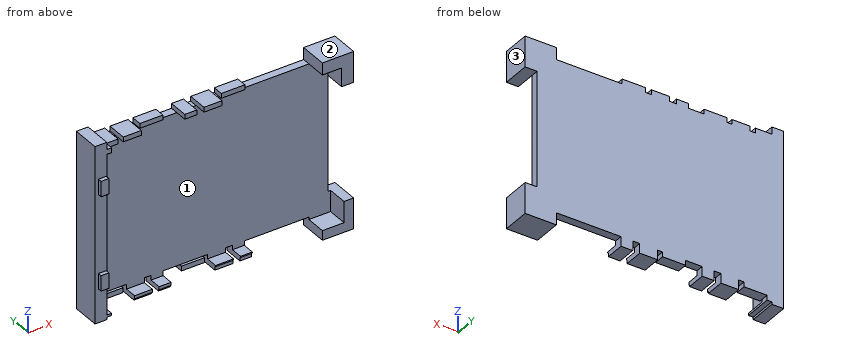
```python
from build123d import *

# Parameters (mm, degrees)
CORNERS_DEPTH                      = 8.4
CORNERS_2_DEPTH                    = 8.4
SKETCH2_W                          = 102.6
SKETCH2_H                          = 63.5
MASTER_DEPTH                       = 3
SKETCH3_W                          = 4.9
SKETCH3_H                          = 73.5
END_TAB_DEPTH                      = 8.36
END_TAB_DEPTH_BACK                 = 3.27
SKETCH4_W                          = 3.2
SKETCH4_H                          = 6.4
MALE_CONNECTORS_DEPTH              = 1.65
SKETCH5_W                          = 9.6
SKETCH5_H                          = 2
SKETCH5_W_2                        = 7.4
SKETCH5_H_2                        = 4
SKETCH5_W_3                        = 5
SKETCH5_W_4                        = 7.5
SKETCH5_W_5                        = 4.9
RIGHT_TERMINALS_DEPTH              = 5
RIGHT_TERMINALS_DEPTH_BACK         = 3.27
SKETCH7_W                          = 4.9
SKETCH7_H                          = 2
LEFT_TERMINALS_DEPTH               = 5
LEFT_TERMINALS_DEPTH_BACK          = 3.27
SKETCH7_W_2                        = 7.5
LEFT_TERMINALS_2_DEPTH             = 5
LEFT_TERMINALS_2_DEPTH_BACK        = 3.27
SKETCH7_W_3                        = 9.6
LEFT_TERMINALS_3_DEPTH             = 5
LEFT_TERMINALS_3_DEPTH_BACK        = 3.27
SKETCH7_W_4                        = 5
LEFT_TERMINALS_4_DEPTH             = 5
LEFT_TERMINALS_4_DEPTH_BACK        = 3.27
LEFT_TERMINALS_5_DEPTH             = 5
LEFT_TERMINALS_5_DEPTH_BACK        = 3.27
SKETCH7_W_5                        = 9.8
LEFT_TERMINALS_6_DEPTH             = 5
LEFT_TERMINALS_6_DEPTH_BACK        = 3.27
SKETCH8_W                          = 9.6
SKETCH8_H                          = 2
GOLD_PLATE_ADJUSTMENTS_RIGHT_DEPTH = 3.9
SKETCH9_W                          = 9.6
SKETCH9_H                          = 2
SKETCH9_W_2                        = 9.8
GOLD_PLATE_ADJUSTMENTS_LEFT_DEPTH  = 3.9
CORNER_ADJUSTMENT_DEPTH            = 3
SKETCH13_W                         = 97.7
SKETCH13_H                         = 63.5
BOSS_EXTRUDE1_DEPTH                = 0.27
SKETCH14_W                         = 13
SKETCH14_H                         = 12.8
BOSS_EXTRUDE2_DEPTH                = 0.27
SKETCH17_W                         = 7.4
SKETCH17_H                         = 2
SKETCH17_W_2                       = 5
SKETCH17_W_3                       = 7.5
SKETCH17_W_4                       = 4.9
CUT_EXTRUDE2_DEPTH                 = 5
SKETCH19_W                         = 15.2
SKETCH19_H                         = 0.4
CUT_EXTRUDE4_DEPTH                 = 0.75
SKETCH20_W                         = 4.9
SKETCH20_H                         = 5
SKETCH20_W_2                       = 7.5
BOSS_EXTRUDE5_DEPTH                = 2.165
SKETCH15_W                         = 2
SKETCH15_H                         = 4
SKETCH15_H_2                       = 2
BOSS_EXTRUDE3_DEPTH                = 11.63
SKETCH21_W                         = 15.3
SKETCH21_H                         = 0.4
CUT_EXTRUDE5_DEPTH                 = 1.65
SKETCH22_W                         = 2
SKETCH22_H                         = 3.074722715
CUT_EXTRUDE7_DEPTH                 = 8.36
SKETCH23_W                         = 9
SKETCH23_H                         = 8.8
CUT_EXTRUDE8_DEPTH                 = 8.4


with BuildPart() as part:
    # Sketch1 → Corners (new body)
    with BuildSketch(Plane(origin=(0, 0, 0), x_dir=(1, 0, 0), z_dir=(0, 1, 0))):
        Polygon((102.6, -63.5), (94.6, -63.5), (94.6, -68.5), (107.6, -68.5), (107.6, -55.7), (102.6, -55.7), align=None)
    extrude(amount=-CORNERS_DEPTH)



with BuildPart() as body_2:
    # Sketch1 → Corners 2 (new body)
    with BuildSketch(Plane(origin=(0, 0, 0), x_dir=(1, 0, 0), z_dir=(0, 1, 0))):
        Polygon((94.6, 5), (94.6, 0), (102.6, 0), (102.6, -7.8), (107.6, -7.8), (107.6, 5), align=None)
    extrude(amount=-CORNERS_2_DEPTH)


with BuildPart() as body_3:
    # Sketch2 → Master (new body)
    with BuildSketch(Plane(origin=(0, 0, 0), x_dir=(1, 0, 0), z_dir=(0, 1, 0))):
        with Locations((51.3, -31.75)):
            Rectangle(SKETCH2_W, SKETCH2_H)
    extrude(amount=MASTER_DEPTH)

    # Sketch3 → End Tab (add, two sides)
    with BuildSketch(Plane.XZ) as end_tab_sk:
        with Locations((2.45, 31.75)):
            Rectangle(SKETCH3_W, SKETCH3_H)
    extrude(amount=END_TAB_DEPTH)
    extrude(end_tab_sk.sketch, amount=-END_TAB_DEPTH_BACK)

    # Sketch4 → Male Connectors (add)
    with BuildSketch(Plane.XZ.offset(8.36)):
        with Locations((3, 12.2)):
            Rectangle(SKETCH4_W, SKETCH4_H)
        with Locations((3, 51.3)):
            Rectangle(SKETCH4_W, SKETCH4_H)
    extrude(amount=MALE_CONNECTORS_DEPTH)

    # Sketch5 → Right Terminals (add, two sides)
    with BuildSketch(Plane.XZ) as right_terminals_sk:
        with Locations((11.7, -1)):
            Rectangle(SKETCH5_W, SKETCH5_H)
        with Locations((22.4, -2)):
            Rectangle(SKETCH5_W_2, SKETCH5_H_2)
        with Locations((31.4, -2)):
            Rectangle(SKETCH5_W_3, SKETCH5_H_2)
        with Locations((45.6, -1)):
            Rectangle(SKETCH5_W, SKETCH5_H)
        with Locations((56.15, -2)):
            Rectangle(SKETCH5_W_4, SKETCH5_H_2)
        with Locations((65.25, -2)):
            Rectangle(SKETCH5_W_5, SKETCH5_H_2)
    extrude(amount=RIGHT_TERMINALS_DEPTH)
    extrude(right_terminals_sk.sketch, amount=-RIGHT_TERMINALS_DEPTH_BACK)

    # Sketch8 → Gold Plate Adjustments (Right) (cut)
    with BuildSketch(Plane.XZ.offset(5)):
        with Locations((11.7, -1)):
            Rectangle(SKETCH8_W, SKETCH8_H)
        with Locations((45.6, -1)):
            Rectangle(SKETCH8_W, SKETCH8_H)
    extrude(amount=-GOLD_PLATE_ADJUSTMENTS_RIGHT_DEPTH, mode=Mode.SUBTRACT)


with BuildPart() as body_4:
    # Sketch7 → Left Terminals (new body, two sides)
    with BuildSketch(Plane.XZ) as left_terminals_sk:
        with Locations((9.35, 64.5)):
            Rectangle(SKETCH7_W, SKETCH7_H)
    extrude(amount=LEFT_TERMINALS_DEPTH)
    extrude(left_terminals_sk.sketch, amount=-LEFT_TERMINALS_DEPTH_BACK)


with BuildPart() as body_5:
    # Sketch7 → Left Terminals 2 (new body, two sides)
    with BuildSketch(Plane.XZ) as left_terminals_2_sk:
        with Locations((17.75, 64.5)):
            Rectangle(SKETCH7_W_2, SKETCH7_H)
    extrude(amount=LEFT_TERMINALS_2_DEPTH)
    extrude(left_terminals_2_sk.sketch, amount=-LEFT_TERMINALS_2_DEPTH_BACK)


with BuildPart() as body_6:
    # Sketch7 → Left Terminals 3 (new body, two sides)
    with BuildSketch(Plane.XZ) as left_terminals_3_sk:
        with Locations((28.3, 64.5)):
            Rectangle(SKETCH7_W_3, SKETCH7_H)
    extrude(amount=LEFT_TERMINALS_3_DEPTH)
    extrude(left_terminals_3_sk.sketch, amount=-LEFT_TERMINALS_3_DEPTH_BACK)


with BuildPart() as body_7:
    # Sketch7 → Left Terminals 4 (new body, two sides)
    with BuildSketch(Plane.XZ) as left_terminals_4_sk:
        with Locations((42.1, 64.5)):
            Rectangle(SKETCH7_W_4, SKETCH7_H)
    extrude(amount=LEFT_TERMINALS_4_DEPTH)
    extrude(left_terminals_4_sk.sketch, amount=-LEFT_TERMINALS_4_DEPTH_BACK)


with BuildPart() as body_8:
    # Sketch7 → Left Terminals 5 (new body, two sides)
    with BuildSketch(Plane.XZ) as left_terminals_5_sk:
        with Locations((51.35, 64.5)):
            Rectangle(SKETCH7_W_2, SKETCH7_H)
    extrude(amount=LEFT_TERMINALS_5_DEPTH)
    extrude(left_terminals_5_sk.sketch, amount=-LEFT_TERMINALS_5_DEPTH_BACK)


with BuildPart() as body_9:
    # Sketch7 → Left Terminals 6 (new body, two sides)
    with BuildSketch(Plane.XZ) as left_terminals_6_sk:
        with Locations((62.3, 64.5)):
            Rectangle(SKETCH7_W_5, SKETCH7_H)
    extrude(amount=LEFT_TERMINALS_6_DEPTH)
    extrude(left_terminals_6_sk.sketch, amount=-LEFT_TERMINALS_6_DEPTH_BACK)


with BuildPart() as gold_plate_adjustments_left_tool:
    # Sketch9 → Gold Plate Adjustments (Left) (new body)
    with BuildSketch(Plane.XZ.offset(5)):
        with Locations((28.3, 64.5)):
            Rectangle(SKETCH9_W, SKETCH9_H)
        with Locations((62.3, 64.5)):
            Rectangle(SKETCH9_W_2, SKETCH9_H)
    extrude(amount=-GOLD_PLATE_ADJUSTMENTS_LEFT_DEPTH)


with BuildPart() as body_6_1:
    add(body_6.part)

    # Gold Plate Adjustments (Left): cut by gold_plate_adjustments_left_tool
    add(gold_plate_adjustments_left_tool.part, mode=Mode.SUBTRACT)


with BuildPart() as body_9_1:
    add(body_9.part)

    # Gold Plate Adjustments (Left): cut by gold_plate_adjustments_left_tool
    add(gold_plate_adjustments_left_tool.part, mode=Mode.SUBTRACT)


with BuildPart() as part_1:
    add(part.part)

    add(body_2.part)  # Corner Adjustment merges body 2

    add(body_3.part)  # Corner Adjustment merges body 3
    # Sketch10 → Corner Adjustment (add)
    with BuildSketch(Plane(origin=(0, 0, 0), x_dir=(1, 0, 0), z_dir=(0, 1, 0))):
        Polygon((102.6, -7.8), (107.6, -7.8), (107.6, 5), (94.6, 5), (94.6, 0), (102.6, 0), align=None)
        Polygon((102.6, -55.7), (107.6, -55.7), (107.6, -68.5), (94.6, -68.5), (94.6, -63.5), (102.6, -63.5), align=None)
    extrude(amount=CORNER_ADJUSTMENT_DEPTH)


    add(body_4.part)  # Boss-Extrude1 merges body 4

    add(body_5.part)  # Boss-Extrude1 merges body 5

    add(body_6_1.part)  # Boss-Extrude1 merges body 6

    add(body_7.part)  # Boss-Extrude1 merges body 7

    add(body_8.part)  # Boss-Extrude1 merges body 8

    add(body_9_1.part)  # Boss-Extrude1 merges body 9
    # Sketch13 → Boss-Extrude1 (add)
    with BuildSketch(Plane(origin=(0, 3, 0), x_dir=(1, 0, 0), z_dir=(0, 1, 0))):
        with Locations((53.75, -31.75)):
            Rectangle(SKETCH13_W, SKETCH13_H)
    extrude(amount=BOSS_EXTRUDE1_DEPTH)

    # Sketch14 → Boss-Extrude2 (add)
    with BuildSketch(Plane(origin=(0, 3, 0), x_dir=(1, 0, 0), z_dir=(0, 1, 0))):
        with Locations((101.1, -62.1)):
            Rectangle(SKETCH14_W, SKETCH14_H)
        with Locations((101.1, -1.4)):
            Rectangle(SKETCH14_W, SKETCH14_H)
    extrude(amount=BOSS_EXTRUDE2_DEPTH)

    # Sketch17 → Cut-Extrude2 (cut)
    with BuildSketch(Plane.XZ.offset(5)):
        with Locations((22.4, -1)):
            Rectangle(SKETCH17_W, SKETCH17_H)
        with Locations((31.4, -1)):
            Rectangle(SKETCH17_W_2, SKETCH17_H)
        with Locations((56.15, -1)):
            Rectangle(SKETCH17_W_3, SKETCH17_H)
        with Locations((65.25, -1)):
            Rectangle(SKETCH17_W_4, SKETCH17_H)
    extrude(amount=-CUT_EXTRUDE2_DEPTH, mode=Mode.SUBTRACT)

    # Sketch19 → Cut-Extrude4 (cut)
    with BuildSketch(Plane(origin=(0, 0, -4), x_dir=(-1, 0, 0), z_dir=(0, 0, -1))):
        with Locations((-26.3, -4.8)):
            Rectangle(SKETCH19_W, SKETCH19_H)
    extrude(amount=-CUT_EXTRUDE4_DEPTH, mode=Mode.SUBTRACT)

    # Sketch20 → Boss-Extrude5 (add)
    with BuildSketch(Plane(origin=(0, 0, -4), x_dir=(-1, 0, 0), z_dir=(0, 0, -1))):
        with Locations((-65.25, -2.5)):
            Rectangle(SKETCH20_W, SKETCH20_H)
        with Locations((-56.15, -2.5)):
            Rectangle(SKETCH20_W_2, SKETCH20_H)
    extrude(amount=-BOSS_EXTRUDE5_DEPTH)

    # Sketch15 → Boss-Extrude3 (add)
    with BuildSketch(Plane(origin=(0, 3.27, 0), x_dir=(1, 0, 0), z_dir=(0, 1, 0))):
        with Locations((5.9, 2)):
            Rectangle(SKETCH15_W, SKETCH15_H)
        with Locations((5.9, -64.5)):
            Rectangle(SKETCH15_W, SKETCH15_H_2)
    extrude(amount=-BOSS_EXTRUDE3_DEPTH)

    # Sketch21 → Cut-Extrude5 (cut)
    with BuildSketch(Plane(origin=(0, 0, -4), x_dir=(-1, 0, 0), z_dir=(0, 0, -1))):
        with Locations((-60.05, -4.8)):
            Rectangle(SKETCH21_W, SKETCH21_H)
    extrude(amount=-CUT_EXTRUDE5_DEPTH, mode=Mode.SUBTRACT)

    # Sketch22 → Cut-Extrude7 (cut)
    with BuildSketch(Plane.XZ.offset(8.36)):
        with Locations((5.9, -1.537361358)):
            Rectangle(SKETCH22_W, SKETCH22_H)
    extrude(amount=-CUT_EXTRUDE7_DEPTH, mode=Mode.SUBTRACT)

    # Sketch23 → Cut-Extrude8 (cut)
    with BuildSketch(Plane.XZ.offset(8.4)):
        with Locations((99.1, 3.4)):
            Rectangle(SKETCH23_W, SKETCH23_H)
    extrude(amount=-CUT_EXTRUDE8_DEPTH, mode=Mode.SUBTRACT)


solid = part_1.part
```
The listing builds one solid part. Answer for the finished solid, in the listing's coordinates (mm). Face numbers are marked on the shaded views. Coordinates: 2 decimals unless noted, no trailing zeros. Loops run counter-clockwise (first coordinate to the right, second up) from the corner with the lowest first, then second, coordinate; pieces in that order, holes last. Notation, with made-up numbers: M 68.25,82.25 L 74.25,82.25 A21 ccw 74.25,105.25 Z; hole C 32.25,-32.75 d10. An arc over 180 degrees is marked long. Answer as CSV lines item,"result". Start each with the question number.
(1) The part is cut by section A-A (z = 4.5). Give the vertices of the cut face in (x, y), and give its area (3 significant figures).
(2) The part is cut by section D-D (z = 29.5). Give the vertices of the cut face in (x, y).
(3) The mould has two halves that part along Z. Classify the marked faces 1, 2 and 3: pulls with the +Z half, pulls with the -Z half, needs draft (parallel to the pull), parting line crosses it, or undercut.
(4) Given pin 1 (2.5 mm diameter, centred on x = 31.5, y = 0, fed in from -Z); pin 2 (5.5 mm diameter, centred on x = 41.5, y = -0.5, fed in from +Z); pin 3 (6 mm diameter, centred on x = 41, z = 5, fed in from -Y), each flat-ended and moving along its own axis, determine where each tip first touches the part or whether it passes through.
(5) The part is cut by section B-B (x = 97). Give the vertices of the cut face in (y, z), and give its area (3 significant figures).
(6) Find the intervals of material crossed by L1, parallel to Y at x = 101, z = 56.5; L2, parallel to X at y = -6.25, z = 39; L3, parallel to X at y = 2.5, z = 55, in increasing order. Write a range as [from, to].
(7) The part is cut by section C-C (y = -2.25). State how many separate pieces and enclosed holes the cut face has, and give its area (3 significant figures).
Determined:
1,outline,"M 0,-8.36 L 4.9,-8.36 L 4.9,0 L 103.6,0 L 103.6,-8.4 L 107.6,-8.4 L 107.6,3.27 L 0,3.27 Z"
1,area,"426 mm2"
2,outline,"M 0,-8.36 L 4.9,-8.36 L 4.9,0 L 102.6,0 L 102.6,3.27 L 0,3.27 Z"
3,face 1,"undercut"
3,face 2,"pulls with the +Z half"
3,face 3,"needs draft"
4,pin 1,"z = -4"
4,pin 2,"z = 65.5"
4,pin 3,"y = 0"
5,outline,"M -8.4,-5 L 3.27,-5 L 3.27,68.5 L -8.4,68.5 L -8.4,63.5 L 0,63.5 L 0,-1 L -8.4,-1 Z"
5,area,"316 mm2"
6,L1,"[0, 3.27]"
6,L2,"[0, 4.9]"
6,L3,"[0, 102.6]"
7,separate pieces,"10"
7,enclosed holes,"0"
7,area,"659 mm2"
